```python
from build123d import *

# Parameters (mm, degrees)
F1_ANGLE_BACK = 30
F1_ANGLE      = 60
F3_DEPTH      = 20
F5_DEPTH      = 20
F6_R          = 1
F7_R          = 1
F8_R          = 1
F9_R          = 1


with BuildPart() as f1:
    # F0 (on Top) → F1 (revolve)
    with BuildSketch(Plane.XY, mode=Mode.PRIVATE) as f1_sk:
        Polygon((-6.7, 15.2109679412), (-9.7, 15.2109679412), (-9.7, -10.7890320588), (-6.7, -10.7890320588), (-6.7, 13.2109679412), (-4.5, 13.2109679412), (-4.5, 3.2109679412), (-2, 3.2109679412), (-2, 13.2109679412), (-2, 15.2109679412), align=None)
    revolve(f1_sk.sketch.rotate(Axis((0, 4.1356552392, 0), (0, -1, 0)), -F1_ANGLE_BACK), axis=Axis((0, 4.1356552392, 0), (0, -1, 0)), revolution_arc=F1_ANGLE)

    # F2 (on face) → F3 (join)
    with BuildSketch(Plane(origin=(0, 0, 0), x_dir=(0.8660254038, 0, -0.5), z_dir=(0.5, 0, 0.8660254038))):
        Polygon((-2, 15.2109679412), (-9.7, 15.2109679412), (-9.7, -10.7890320588), (-6.7, -10.7890320588), (-6.7, 13.2109679412), (-4.5, 13.2109679412), (-4.5, 3.2109679412), (-2, 3.2109679412), align=None)
    extrude(amount=F3_DEPTH)

    # F4 (on face) → F5 (join)
    with BuildSketch(Plane(origin=(0, 0, 0), x_dir=(0.8660254038, 0, 0.5), z_dir=(0.5, 0, -0.8660254038))):
        Polygon((-2, -15.2109679412), (-2, -3.2109679412), (-4.5, -3.2109679412), (-4.5, -13.2109679412), (-6.7, -13.2109679412), (-6.7, 10.7890320588), (-9.7, 10.7890320588), (-9.7, -15.2109679412), align=None)
    extrude(amount=F5_DEPTH)

    # F6
    f6_edges = [f1.edges().sort_by_distance(p)[0] for p in [
        (1.102886, 3.210968, 10.910254),
        (-3.400446, 15.210968, -13.510254),
    ]]
    fillet(f6_edges, radius=F6_R)

    # F7
    f7_edges = [f1.edges().sort_by_distance(p)[0] for p in [
        (3.267949, 15.210968, -9.660254),
    ]]
    fillet(f7_edges, radius=F7_R)

    # F8
    f8_edges = [f1.edges().sort_by_distance(p)[0] for p in [
        (4.933751, 15.210968, 20.245508),
    ]]
    fillet(f8_edges, radius=F8_R)

    # F9
    f9_edges = [f1.edges().sort_by_distance(p)[0] for p in [
        (1.599554, 1.710968, -22.170508),
    ]]
    fillet(f9_edges, radius=F9_R)


solid = f1.part
```
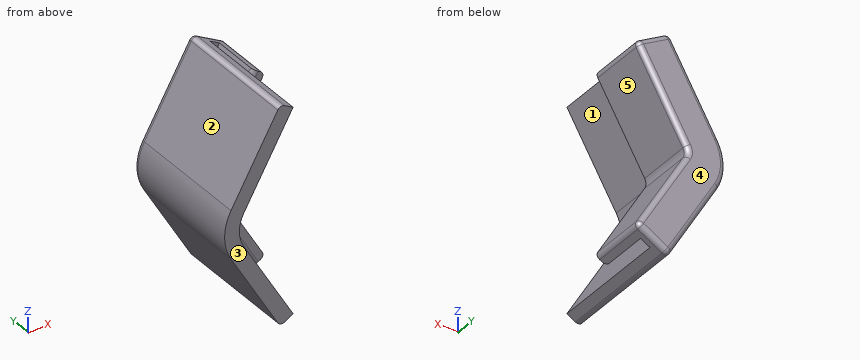
Model file for the job. Use its own axes, mm. Face numbers are marked on the shaded views. A direction names the side the tool comes from. Coordinates: 2 decimals unless noted, no trailing zeros. Loops run counter-clockwise (first coordinate to the right, second up) from the corner with the lowest first, then second, coordinate; pieces in that order, holes last. Notation, with made-up numbers: M 12,22.5 L 33,22.5 A15 cw 33,42.5 Z; hole C 83.25,29 d8. An arc over 180 degrees is marked long. Use CSV: the item, a comma, the result in double quotes. Start each with the question number.
1. Band-saw the part on A-A, the plane y = 11. List the corners of the cut face in (x, z).
2. Band-saw the part on C-C, the plane y = -5.5. List the corners of the cut face in (x, z).
3. Two-plate mould, pull along Z, no slides. Class the marked faces 1, 2 and 3: pulls with the +Z half, pulls with the -Z half, needs draft (parallel to the pull), parting line crosses it, or undercut.
4. Tool access for the marked faces 4 and 5: list every direction of +Z, -Z, +X, -X, +Y, -Y with a clear straight run to the whole face (end or side of a thin tool).
5. Probe probe 1 along Z at (x, y) = (0.75, 8.5); probe 2 along X at (y, z) = (3.5, -12.5); probe 3 along X at (y, z) = (11.75, -5). List the from-to ranges inside material, lowest first. Write a range as [from, to].
6. Flat gauge pins, fed straight in: pin 1 (2 mm diameter, centred on x = 4.5, y = 11, fed in from +Z); pin 2 (4 mm diameter, centred on y = 8, z = 8, fed in from +X); pin 3 (1.5 mm diameter, centred on y = -2, z = 13, fed in from +X). Where does each tip first touch, or does it go through?
7. Band-saw the part on B-B, the plane z = 0. List the corners of the cut face in (x, y).
Entries:
1,outline,"M -8.4,-4.85 L 1.1,-21.3 A1 ccw 2.47,-21.67 L 4.2,-20.67 L -5.8,-3.35 A6.7 cw -5.8,3.35 L 4.2,20.67 L 2.47,21.67 A1 ccw 1.1,21.3 L -8.4,4.85 A9.7 ccw Z; M -3.9,-2.25 L 6.1,-19.57 L 7.4,-18.82 A1 ccw 7.77,-17.45 L -1.73,-1 A2 cw -1.73,1 L 7.77,17.45 A1 ccw 7.4,18.82 L 6.1,19.57 L -3.9,2.25 A4.5 ccw Z"
2,outline,"M -8.4,-4.85 L 1.1,-21.3 A1 ccw 2.47,-21.67 L 4.2,-20.67 L -5.8,-3.35 A6.7 cw -5.8,3.35 L 4.2,20.67 L 2.47,21.67 A1 ccw 1.1,21.3 L -8.4,4.85 A9.7 ccw Z"
3,face 1,"undercut"
3,face 2,"pulls with the +Z half"
3,face 3,"needs draft"
4,face 4,"+Z, -Z, +X, -X, +Y"
4,face 5,"+X, +Y, -Y"
5,probe 1,"z = [-20.7, -14.7], [-10.3, -5.3], [5.3, 10.3], [14.7, 20.7]"
5,probe 2,"x = [-3.98, -0.52], [2.36, 4.91]"
5,probe 3,"x = [-8.31, -4.85], [-2.31, 0.58]"
6,pin 1,"stops at z = 21.07"
6,pin 2,"stops at x = 3.46"
6,pin 3,"stops at x = 0.2"
7,outline,"M -9.7,-10.79 L -6.7,-10.79 L -6.7,13.21 L -4.5,13.21 L -4.5,4.21 A1 ccw -3.5,3.21 L -2,3.21 L -2,14.21 A1 ccw -3,15.21 L -8.7,15.21 A1 ccw -9.7,14.21 Z"
